Verification items for the finished model (mm, model axes). A direction names the side the tool comes from. Give positions to 0.01 mm unless a question says otherwise; leave off trailing zeros. Order: outer loops, then holes, each group sorted by start corner. A loop starts at its lowest first (then second) coordinate and runs counter-clockwise, first axis right, second up.
from build123d import *

# Parameters (mm, degrees)
SKETCH_R      = 30
SKETCH_R_2    = 21
PAD_DEPTH     = 4
SKETCH001_R   = 25
SKETCH001_R_2 = 21
PAD001_DEPTH  = 24
SKETCH002_R   = 25
SKETCH002_R_2 = 21
PAD002_DEPTH  = 10


with BuildPart() as part:
    # Sketch → Pad (new body)
    with BuildSketch(Plane.XY):
        Circle(SKETCH_R)
        Circle(SKETCH_R_2, mode=Mode.SUBTRACT)
    extrude(amount=PAD_DEPTH)

    # Sketch001 (on Face3 of Pad) → Pad001 (join)
    with BuildSketch(Plane(origin=(0, 0, 0), x_dir=(1, 0, 0), z_dir=(0, 0, -1))):
        Circle(SKETCH001_R)
        Circle(SKETCH001_R_2, mode=Mode.SUBTRACT)
    extrude(amount=PAD001_DEPTH)

    # Sketch002 (on Face3 of Pad001) → Pad002 (join)
    with BuildSketch(Plane.XY.offset(4)):
        Circle(SKETCH002_R)
        Circle(SKETCH002_R_2, mode=Mode.SUBTRACT)
    extrude(amount=PAD002_DEPTH)


solid = part.part
(1) Section check C-C, the plane z = 9. Enter the section's corners in (x, y), then the cut area to 3 significant figures.
Solved:
outline: circle Ø50 at (0, 0); hole circle Ø42 at (0, 0)
area: 578 mm2
(2) Release check for a two-part mould opening along X. For faces 1 (the cylindrical face through (20.03, 6.31, -5.27)), 2 (the cylindrical face through (23.846, 7.509, 8.93)), 3 (the flat face through (-7, 25, 0)) record: pulls with the +X half, pulls with the -X half, needs draft (parallel to the pull), parting line crosses it, or undercut.
Solved:
face 1: undercut
face 2: parting line crosses it
face 3: needs draft
(3) Section check A-A, the plane x = 0. Enter the section's corners in (y, z), then the cut area to 3 significant figures.
Solved:
outline: (-30, 0) - (-25, 0) - (-25, -24) - (-21, -24) - (-21, 14) - (-25, 14) - (-25, 4) - (-30, 4) - close; (21, -24) - (25, -24) - (25, 0) - (30, 0) - (30, 4) - (25, 4) - (25, 14) - (21, 14) - close
area: 344 mm2
(4) Scan lines: line 1 (X direction, y = 0, z = -2); line 2 (Y direction, x = 15, z = -8.5). Record each from-to range of solid material in increasing order.
Solved:
line 1: x = -25 to -21, 21 to 25
line 2: y = -20 to -14.7, 14.7 to 20
(5) Set-up check for faces 4 (the cylindrical face through (-29.97, 1.32, 1.97)), 5 (the cylindrical face through (23.846, -7.509, -11.832)), 6 (the flat face through (-7, 25, 4)): record each of +Z, -Z, +X, -X, +Y, -Y from which the full face is reachable in a straight line by a thin tool's end or side.
Solved:
face 4: +Z, -Z
face 5: -Z
face 6: +Z
(6) Go/stop test with flat-tipped pins: pin 1 (10 mm diameter, centred on y = 8, z = -12, fed in from -X); pin 2 (1.5 mm diameter, centred on y = -15.5, z = -2, fed in from -X); pin 3 (5 mm diameter, centred on x = 5, y = 15.5, fed in from -Z); pin 4 (4 mm diameter, centred on y = 18.5, z = -4, fed in from +X). Record where each tip stops, or that it passes through.
Solved:
pin 1: stops at x = -24.82
pin 2: stops at x = -20.19
pin 3: passes through
pin 4: stops at x = 18.78
